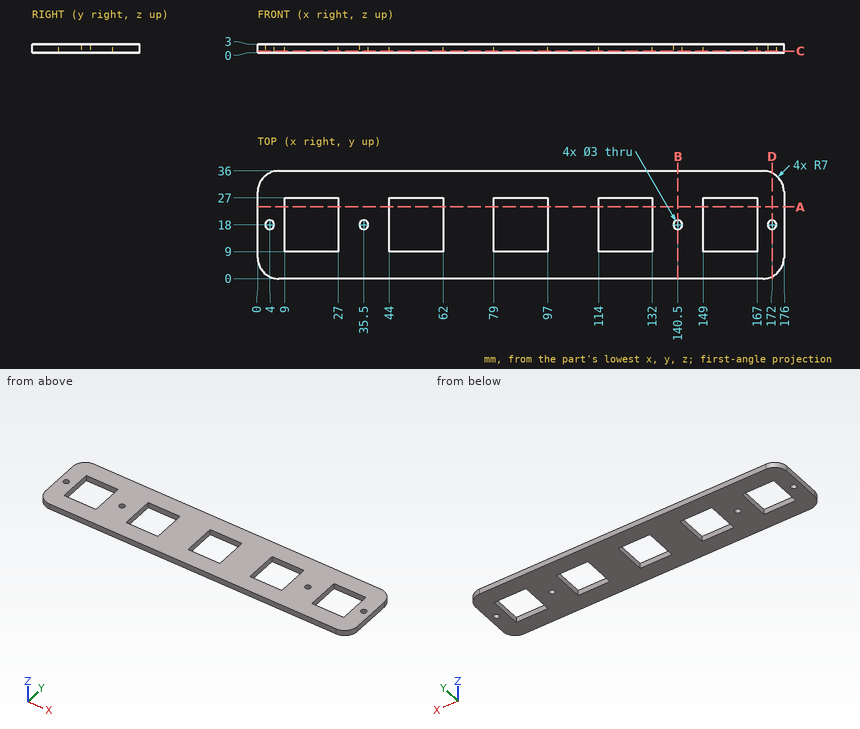
Geometry: see drawing. Coordinates: mm, zero at the bounding-box minimum. Round coordinates to 2 decimals unless told otherwise and drop trailing zeros. Loops run counter-clockwise (first coordinate to the right, second up) from the corner with the lowest first, then second, coordinate; pieces in that order, holes last. Notation, with made-up numbers: M 20,-18.5 L 41,-18.5 A29 ccw 41,9.5 Z; hole C 4.25,20 d1. An arc over 180 degrees is marked long. Use a Markdown table: item, result. Add a question column.
1. Ray query, line 1 along X through (y, z) = (10, 1.55); line 2 along Y through (x, z) = (80.5, 0.9); line 3 along Y through (x, z) = (35.5, 1.65). Return the intervals inside material, ascending. Write a range as [from, to].
2. Cut plane B-B, the plane x = 140.5. Output: boundary loops of the cut face in (y, z).
3. Cut plane A-A, the plane y = 24. Output: boundary loops of the cut face in (x, z).
4. Cut plane D-D, the plane x = 172. Output: boundary loops of the cut face in (y, z), and give its area (3 significant figures).
5. Cut plane C-C, the plane z = 0.6. State how many separate pieces and enclosed holes the cut face has, and give its area (3 significant figures).
Solution:
| question | item | result |
|---|---|---|
| 1 | line 1 | x = [0, 9], [27, 44], [62, 79], [97, 114], [132, 149], [167, 176] |
| 1 | line 2 | y = [0, 9], [27, 36] |
| 1 | line 3 | y = [0, 16.5], [19.5, 36] |
| 2 | outline | M 0,0 L 16.5,0 L 16.5,3 L 0,3 Z; M 19.5,0 L 36,0 L 36,3 L 19.5,3 Z |
| 3 | outline | M 0,0 L 9,0 L 9,3 L 0,3 Z; M 27,0 L 44,0 L 44,3 L 27,3 Z; M 62,0 L 79,0 L 79,3 L 62,3 Z; M 97,0 L 114,0 L 114,3 L 97,3 Z; M 132,0 L 149,0 L 149,3 L 132,3 Z; M 167,0 L 176,0 L 176,3 L 167,3 Z |
| 4 | outline | M 0.68,0 L 16.5,0 L 16.5,3 L 0.68,3 Z; M 19.5,0 L 35.32,0 L 35.32,3 L 19.5,3 Z |
| 4 | area | 94.9 mm2 |
| 5 | separate pieces | 1 |
| 5 | enclosed holes | 9 |
| 5 | area | 4,650 mm2 |
